```python
from build123d import *

# Parameters (mm, degrees)
F1_DEPTH = 70
F2_R     = 3.25
F3_DEPTH = 2
F4_R     = 2.1
F5_DEPTH = 4


with BuildPart() as f1:
    # F0 (on Front) → F1 (new body)
    with BuildSketch(Plane.XZ):
        Polygon((49.424573, 12.242154), (49.424573, 27.742154), (43.424573, 23.742154), (43.424573, 16.242154), align=None)
    extrude(amount=F1_DEPTH)

    # F2 (on face) → F3 (cut)
    with BuildSketch(Plane.YZ.offset(49.424573)):
        with Locations((-65, 19.992154)):
            Circle(F2_R)
        with Locations((-5, 19.992154)):
            Circle(F2_R)
    extrude(amount=-F3_DEPTH, mode=Mode.SUBTRACT)

    # F4 (on face) → F5 (cut)
    with BuildSketch(Plane(origin=(43.424573, 0, 0), x_dir=(0, -1, 0), z_dir=(-1, 0, 0))):
        with Locations((5, 19.992154)):
            Circle(F4_R)
        with Locations((65, 19.992154)):
            Circle(F4_R)
    extrude(amount=-F5_DEPTH, mode=Mode.SUBTRACT)


solid = f1.part
```
Input: part model. Units: mm. Frame: model coordinates. A direction names the side the tool comes from. Round coordinates to 2 decimals unless told otherwise and drop trailing zeros. Loops run counter-clockwise (first coordinate to the right, second up) from the corner with the lowest first, then second, coordinate; pieces in that order, holes last. Notation, with made-up numbers: (-19, -21.75) -> (-10, -21.75) arc R11 ccw to (-10, -8.75) -> close; hole circle Ø4 at (61.5, 19.5). An arc over 180 degrees is marked (long way). Write each question's results on one line, items separated by ' | '.
1. Section C-C (y = -13.5). Return loops of the section in (x, z).
Geometry results:
outline: (43.42, 16.24) -> (49.42, 12.24) -> (49.42, 27.74) -> (43.42, 23.74) -> close
2. Section B-B (x = 46.65). Return loops of the section in (y, z).
Geometry results:
outline: (-70, 14.09) -> (0, 14.09) -> (0, 25.89) -> (-70, 25.89) -> close; hole circle Ø4.2 at (-65, 19.99); hole circle Ø4.2 at (-5, 19.99)
3. Set-up query: faces 4 (the face through (47, 0, 20)), 5 (the face through (47.425, -2.9, 20.8)). Return all of +Z, -Z, +X, -X, +Y, -Y with unobstructed straight access to the full face (end or side cutting, diameter ignored); none if empty.
Geometry results:
face 4: +Z, -Z, +X, -X, +Y | face 5: +X
4. Mould query, pull axis Z, two halves, no side actions, for faces 1 (the face through (48.439, -5.423, 23.214)), 2 (the face through (47, -70, 20)), 3 (the face through (46.467, -34.51, 25.77)). Classes: +Z half, -Z half, draft (parallel to the pull), parting line (faces both ways), or undercut.
Geometry results:
face 1: undercut | face 2: draft | face 3: +Z half
5. Section D-D (z = 14.5). Return loops of the section in (x, y), and give its area (3 significant figures).
Geometry results:
outline: (46.04, -70) -> (49.42, -70) -> (49.42, 0) -> (46.04, 0) -> close | area: 237 mm2
6. Ray query, line 1 (Z direction, x = 45.5, y = -65.5); line 2 (Z direction, x = 48.95, y = -65); line 3 (Z direction, x = 44.15, y = -17.5). Return the intervals inside material, ascending. Write a range as from..to.
Geometry results:
line 1: 14.86..17.95, 22.03..25.13 | line 2: 12.56..16.74, 23.24..27.43 | line 3: 15.76..24.23
7. First-contact query: P1, Ø1.5, axis at x = 45, y = -21.5, coming from the -Z side; P2, Ø5, axis at y = -65, z = 19.99, coming from the +X side. Flat tips, straight axial feed; report the tip coordinate or a pass-through.
Geometry results:
P1: z = 14.69 | P2: x = 47.42
8. Section A-A (y = -65). Return loops of the section in (x, z).
Geometry results:
outline: (43.42, 16.24) -> (49.42, 12.24) -> (49.42, 16.74) -> (47.42, 16.74) -> (47.42, 17.89) -> (43.42, 17.89) -> close; (43.42, 22.09) -> (47.42, 22.09) -> (47.42, 23.24) -> (49.42, 23.24) -> (49.42, 27.74) -> (43.42, 23.74) -> close
